```python
from build123d import *

# Parameters (mm, degrees)
F2_T = -2.5
F4_D = 20


with BuildPart() as f1:
    # F0 (on Right) → F1 (revolve)
    with BuildSketch(Plane.YZ):
        Polygon((-50, 0), (0, 0), (0, 282.842712), (-150, 282.842712), align=None)
    revolve(axis=Axis((0, 0, 141.421356), (0, 0, -1)))

    # F2
    f2_openings = [f1.faces().sort_by_distance(p)[0] for p in [
        (0, 0, 282.842712),
    ]]
    offset(amount=F2_T, openings=f2_openings)

    # F4 (through all)
    with Locations(Plane(origin=(0, 0, 0), x_dir=(1, 0, 0), z_dir=(0, 0, -1))):
        with Locations((0, 0)):
            Hole(F4_D / 2)


solid = f1.part
```
Check sheet for the modelled part. Datum: model origin and axes. Units: mm. A direction names the side the tool comes from. Round coordinates to 2 decimals unless told otherwise and drop trailing zeros. Order: outer loops, then holes, each group sorted by start corner. A loop starts at its lowest first (then second) coordinate and runs counter-clockwise, first axis right, second up. Notation, with made-up numbers: (74.25, -15) - (123.25, -15) arc R21 cw to (123.25, 9) - close; hole circle Ø8 at (27, 51). An arc over 180 degrees is marked (long way). Write item = value, one per line.
Q1. Section check D-D (z = 136). Record the boundary of the cut face in (x, y), and give its area (3 significant figures).
Computed:
outline = circle Ø196.17 at (0, 0); hole circle Ø190.86 at (0, 0)
area = 1,610 mm^2
Q2. Section check A-A (y = 0). Record the boundary of the cut face in (x, z).
Computed:
outline = (-150, 282.84) - (-50, 0) - (-10, 0) - (-10, 2.5) - (-48.23, 2.5) - (-147.35, 282.84) - close; (10, 0) - (50, 0) - (150, 282.84) - (147.35, 282.84) - (48.23, 2.5) - (10, 2.5) - close
Q3. Thickness scan on line 1 along Z through (x, y) = (25, -39); line 2 along X through (y, z) = (48, 253); line 3 along X through (y, z) = (84, 200.5). Record the ranges inside material, lowest first.
Computed:
line_1 = 0 to 2.5
line_2 = -130.93 to -128.1, 128.1 to 130.93
line_3 = -86.94 to -83.21, 83.21 to 86.94
Q4. Section check C-C (z = 23.5). Record the boundary of the cut face in (x, y).
Computed:
outline = circle Ø116.62 at (0, 0); hole circle Ø111.31 at (0, 0)
Q5. Draft check along X on faces 1 (the face through (78.24, -40.69, 108.01)), 2 (the face through (76.4, -39.7, 109.6)), 3 (the face through (10.4, 0.7, 0)). Enter one of: pulls with the +X half, pulls with the -X half, needs draft (parallel to the pull), parting line crosses it, or undercut.
Computed:
face_1 = parting line crosses it
face_2 = undercut
face_3 = needs draft
Q6. Go/stop test with flat-tipped pins: pin 1 (6 mm diameter, centred on x = 25, y = 13, fed in from +Z); pin 2 (6 mm diameter, centred on x = 119, z = 239, fed in from +Y); pin 3 (10 mm diameter, centred on x = 58.5, z = 201.5, fed in from +Y). Record where each tip stops, or that it passes through.
Computed:
pin_1 = 2.5
pin_2 = 68.49
pin_3 = 109.49
Q7. Tool access check on faces 4 (the face through (-11, 1, 2.5)), 5 (the face through (2.17, 9.76, 1.27)). Record the directions out of +Z, -Z, +X, -X, +Y, -Y that give a thin tool (end or side, any length) a straight path to the whole face; none if there is none.
Computed:
face_4 = +Z
face_5 = +Z, -Z
